Autodesk Inventor part; units mm, degrees
ref_plane "YZ Plane" through (0, 0, 0) normal (1, 0, 0) x (0, 1, 0)
ref_plane "XZ Plane" through (0, 0, 0) normal (0, 1, 0) x (-1, 0, 0)
ref_plane "XY Plane" through (0, 0, 0) normal (0, 0, 1) x (1, 0, 0)
sketch "Sketch1" plane through (0, 0, 0) normal (0, 0, 1) x (1, 0, 0)
  line L0 (-44.45, 19.05) -> (44.45, 19.05)
  line L1 (44.45, 19.05) -> (44.45, -19.05)
  line L2 (44.45, -19.05) -> (-44.45, -19.05)
  line L3 (-44.45, -19.05) -> (-44.45, 19.05)
  line L4 (-44.45, 19.05) -> (44.45, -19.05) construction
  line L5 (44.45, 19.05) -> (-44.45, -19.05) construction
  point P0 (0, 0)
  dimension "d0" = 88.9
  dimension "d1" = 38.1
extrude "Extrusion1" add sketch "Sketch1" along normal blind 355.6
chamfer "Chamfer1" distance 38.1 angle 45 2 edges at (0, 19.05, 355.6) (0, 19.05, 0)
fillet "Fillet1" radius 3.175 4 edges at (-44.45, 19.05, 177.8) (-44.45, -19.05, 177.8) (44.45, -19.05, 177.8) (44.45, 19.05, 177.8)
properties part number "Upper Decoration"
Work out the finished part from the listing and answer in its coordinate system (mm). Coordinates: 2 decimals unless noted, no trailing zeros. Write each loop counter-clockwise with the first axis right and the second up, starting at its lowest first coordinate (ties: lowest second). Pieces come first, ordered by that corner, then holes.
Q1. A cutting plane is placed at B-B, the plane y = -3. Give the vertices of the cut face in (x, z).
Q2. Each of these flat-tipped pins is pushed along its axis until it touches: pin 1 Ø8 at (x, y) = (20, -14) entering from +Z; pin 2 Ø1.5 at (x, y) = (7.5, 4.5) entering from +Z; pin 3 Ø12 at (x, y) = (-20, -13) entering from -Z. Where does it stop, or does it pass through?
Q3. A cutting plane is placed at C-C, the plane y = 10. Give the vertices of the cut face in (x, z), then the cut area to 3 significant figures.
Q4. Find the intervals of material crossed by line 1 (Z direction, x = 28, y = 14); line 2 (Z direction, x = 26, y = -6), in increasing order.
Findings below:
1. outline: (-44.45, 16.05) - (44.45, 16.05) - (44.45, 339.55) - (-44.45, 339.55) - close
2. pin 1: stops at z = 354.55
2. pin 2: stops at z = 332.8
2. pin 3: stops at z = 0.05
3. outline: (-44.45, 29.05) - (44.45, 29.05) - (44.45, 326.55) - (-44.45, 326.55) - close
3. area: 26,400 mm2
4. line 1: z = 33.05 to 322.55
4. line 2: z = 13.05 to 342.55
